Work out the finished part from the listing and answer in its coordinate system (mm). Face numbers are marked on the shaded views. A direction names the side the tool comes from. Round coordinates to 2 decimals unless told otherwise and drop trailing zeros. Order: outer loops, then holes, each group sorted by start corner. A loop starts at its lowest first (then second) coordinate and runs counter-clockwise, first axis right, second up. Notation, with made-up numbers: (18, -17) -> (47, -17) arc R15 cw to (47, -10) -> close; hole circle Ø10 at (72.25, -11). An arc over 180 degrees is marked (long way). Use a Markdown table: item, result. Add a question column.
Item 1: Find the intervals of material crossed by L1, parallel to Y at x = 0, z = 3.6; L2, parallel to Y at x = -19.5, z = 4.5; L3, parallel to Y at x = -1, z = 4.7, in increasing order. Write a range as [from, to].
Item 2: A tool of negligible diameter and unlimited length cuts with its end or side. For the marked faces 5, 6 and 7, from which of +Z, -Z, +X, -X, +Y, -Y can it reach the whole face along a straight path? Write none if from no direction.
Item 3: A cutting plane is placed at B-B, the plane x = 0. Determine the outline of the cut face in (y, z).
Item 4: Flat-ended cylindrical pins translate along their axes: P1, Ø2.5, axis at x = 13.5, y = -14.5, coming from the -Z side; P2, Ø2.5, axis at x = 0, y = 28, coming from the +Z side; P3, Ø2.5, axis at x = 6.5, z = 1, coming from the +Y side; P4, Ø3, axis at y = -6.5, z = 4, coming from the +X side. Find the tip coordinate at first contact, or state that the pin passes through.
Item 5: A cutting plane is placed at C-C, the plane z = 3.15. Determine the outline of the cut face in (x, y).
Item 6: A cutting plane is placed at A-A, the plane y = 0. Determine the outline of the cut face in (x, z), plus the area to 3 significant figures.
Item 7: A cutting plane is placed at D-D, the plane y = 28. Determine the outline of the cut face in (x, z), plus the area to 3 significant figures.
Item 8: For a pull along Y with two mould halves and no side action, classify the marked faces 1, 2, 3 and 4 as +Y half, -Y half, draft (parallel to the pull), parting line (faces both ways), or undercut.
Autodesk Inventor part; units mm, degrees
ref_plane "YZ Plane" through (0, 0, 0) normal (1, 0, 0) x (0, 1, 0)
ref_plane "XZ Plane" through (0, 0, 0) normal (0, 1, 0) x (-1, 0, 0)
ref_plane "XY Plane" through (0, 0, 0) normal (0, 0, 1) x (1, 0, 0)
sketch "Sketch1" plane through (0, 0, 0) normal (0, 0, 1) x (1, 0, 0)
  circle A0 centre (0, 28) radius 1.6
  circle A1 centre (0, -28) radius 1.6
  arc A2 (-32.9803, -13) -> (32.9803, -13) centre (0, 0) ccw
  arc A3 (32.9803, -13) -> (32.9803, 13) centre (0, 0) ccw
  arc A4 (32.9803, 13) -> (-32.9803, 13) centre (0, 0) ccw
  arc A5 (-32.9803, 13) -> (-32.9803, -13) centre (0, 0) ccw
extrude "Extrusion1" add sketch "Sketch1" along normal blind 5
sketch "Sketch2" plane through (0, 0, 0) normal (0, 0, -1) x (-1, 0, 0)
  line L0 (-35.45, 17.5) -> (35.45, 17.5)
  line L1 (35.45, 17.5) -> (35.45, -17.5)
  line L2 (35.45, -17.5) -> (-35.45, -17.5)
  line L3 (-35.45, -17.5) -> (-35.45, 17.5)
  line L4 (-35.45, 17.5) -> (35.45, -17.5) construction
  line L5 (35.45, 17.5) -> (-35.45, -17.5) construction
  circle A0 centre (0, 0) radius 35.45
  point P0 (-30.8294, 17.5)
  point P1 (-30.8294, -17.5)
  point P2 (30.8294, -17.5)
  point P3 (30.8294, 17.5)
  dimension "d2" = 35
extrude "Extrusion2" cut sketch "Sketch2" against normal blind 0.2 contours L0 A0 L2
sketch "Sketch3" plane through (0, 0, 0.2) normal (0, 0, -1) x (-1, 0, 0)
  line L0 (-20, -13) -> (-20, 13)
  line L1 (-20, 13) -> (20, 13)
  line L2 (20, 13) -> (20, -13)
  line L3 (20, -13) -> (-20, -13)
  circle A0 centre (0, 28) radius 1.6
  circle A1 centre (0, -28) radius 1.6
  circle A2 centre (0, 0) radius 34.25
extrude "Extrusion3" cut sketch "Sketch3" against normal through all contours L0 L1 L2 L3
chamfer "Chamfer1" distance 2 angle 45 2 edges at (-35.45, 0, 0.2) (35.3622, -2.4938, 0.2)
sketch "Sketch4" plane through (0, 0, 0.2) normal (0, 0, -1) x (-1, 0, 0)
  line L0 (-20, 13) -> (20, 13)
  line L1 (20, -13) -> (-20, -13)
  line L2 (-20, -13) -> (-20, 13)
  line L3 (20, 13) -> (20, -13)
  circle A0 centre (0, 0) radius 35.45
  line L4 (20, 13) -> (-20, 13)
  line L5 (-20, 13) -> (-32.9803, 13)
  line L6 (-20, 13) -> (-20, -13)
  line L7 (-20, -13) -> (-32.9803, -13)
  arc A1 (-30.8294, 17.5) -> (-30.8294, -17.5) centre (0, 0) ccw
  line L8 (-20, -13) -> (20, -13)
  line L9 (20, -13) -> (32.9803, -13)
  circle A2 centre (0, 0) radius 35.45
  line L10 (20, -13) -> (20, 13)
  line L11 (20, 13) -> (32.9803, 13)
  point P0 (26.4902, -13)
extrude "Extrusion4" cut sketch "Sketch4" against normal blind 1.3 contours L2 L7 A0 L5 | L11 A0 L9 L3
properties part number "FilmGuide"
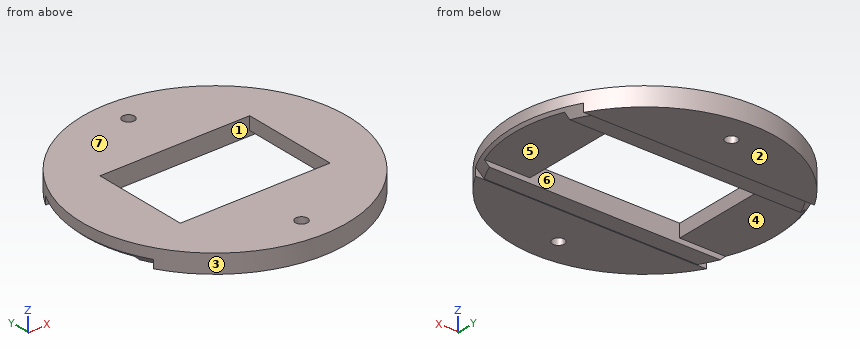
Reported:
| question | item | result |
|---|---|---|
| 1 | L1 | [-35.45, -29.6], [-26.4, -13], [13, 26.4], [29.6, 35.45] |
| 1 | L2 | [-29.6, -13], [13, 29.6] |
| 1 | L3 | [-35.44, -29.25], [-26.75, -13], [13, 26.75], [29.25, 35.44] |
| 2 | face 5 | -Z, +X, -X |
| 2 | face 6 | -Z |
| 2 | face 7 | +Z, +X, -X, +Y, -Y |
| 3 | outline | (-35.45, 0) -> (-29.6, 0) -> (-29.6, 5) -> (-35.45, 5) -> close; (-26.4, 0) -> (-17.5, 0) -> (-17.5, 0.2) -> (-13, 0.2) -> (-13, 5) -> (-26.4, 5) -> close; (13, 0.2) -> (17.5, 0.2) -> (17.5, 0) -> (26.4, 0) -> (26.4, 5) -> (13, 5) -> close; (29.6, 0) -> (35.45, 0) -> (35.45, 5) -> (29.6, 5) -> close |
| 4 | P1 | z = 0.2 |
| 4 | P2 | through |
| 4 | P3 | y = 35.06 |
| 4 | P4 | x = 35.1 |
| 5 | outline | circle Ø70.9 at (0, 0); hole (-20, -13) -> (20, -13) -> (20, 13) -> (-20, 13) -> close; hole circle Ø3.2 at (0, -28); hole circle Ø3.2 at (0, 28) |
| 6 | outline | (-35.45, 2.2) -> (-34.75, 1.5) -> (-20, 1.5) -> (-20, 5) -> (-35.45, 5) -> close; (20, 1.5) -> (34.75, 1.5) -> (35.45, 2.2) -> (35.45, 5) -> (20, 5) -> close |
| 6 | area | 108 mm² |
| 7 | outline | (-21.74, 0) -> (-1.6, 0) -> (-1.6, 5) -> (-21.74, 5) -> close; (1.6, 0) -> (21.74, 0) -> (21.74, 5) -> (1.6, 5) -> close |
| 7 | area | 201 mm² |
| 8 | face 1 | undercut |
| 8 | face 2 | draft |
| 8 | face 3 | parting line |
| 8 | face 4 | undercut |
